```python
from build123d import *

# Parameters (mm, degrees)
SKETCH1_R           = 35
SKETCH1_R_2         = 15
BOSS_EXTRUDE1_DEPTH = 10
SKETCH5_R           = 35
BOSS_EXTRUDE3_DEPTH = 10
SKETCH4_R           = 2.5
BOSS_EXTRUDE2_DEPTH = 2


with BuildPart() as part:
    # Sketch1 → Boss-Extrude1 (new body)
    with BuildSketch(Plane.XY):
        Circle(SKETCH1_R)
        Circle(SKETCH1_R_2, mode=Mode.SUBTRACT)
    extrude(amount=BOSS_EXTRUDE1_DEPTH)

    # Sketch2 for Loft1 → Loft1 section 0
    with BuildSketch(Plane(origin=(0, 0, 0), x_dir=(0, 0, -1), z_dir=(1, 0, 0))):
        with BuildLine():
            Line((-10, -20), (-2.996710384, -20))
            # circular arc as an exact rational Bezier (weights 1, cos(half-angle), 1)
            Bezier((-2.996710384, -20), (35, -55.538461538), (72.996710384, -20), weights=[1, 0.730337079, 1])
            Line((72.996710384, -20), (80, -20))
            Bezier((80, -20), (35, -69.846153846), (-10, -20), weights=[1, 0.670103093, 1])
        make_face()
    # Sketch3 for Loft1 → Loft1 section 1
    with BuildSketch(Plane(origin=(100, 0, 0), x_dir=(0, 0, -1), z_dir=(1, 0, 0))):
        with BuildLine():
            Line((10, -15), (6.551180448, -15))
            Bezier((6.551180448, -15), (40, -77.258592471), (73.448819552, -15), weights=[1, 0.47327653, 1])
            Line((73.448819552, -15), (70, -15))
            Bezier((70, -15), (40, -65.081833061), (10, -15), weights=[1, 0.513877208, 1])
        make_face()
    loft()

    # Sketch5 → Boss-Extrude3 (add)
    with BuildSketch(Plane.XY.offset(10)):
        with Locations(Location((0, 0, 0), (0, 0, 314.528269686))):
            Circle(SKETCH5_R)
    extrude(amount=BOSS_EXTRUDE3_DEPTH)

    # Sketch7 → Revolve1 (revolve)
    with BuildSketch(Plane.ZY, mode=Mode.PRIVATE) as revolve1_sk:
        with BuildLine():
            Line((20, 34), (20, 39))
            Line((20, 39), (17.5, 39))
            Line((17.5, 39), (16.153846154, 35.769230769))
            ThreePointArc((16.153846154, 35.769230769), (15, 35), (13.846153846, 35.769230769))
            Line((13.846153846, 35.769230769), (12.5, 39))
            Line((12.5, 39), (10, 39))
            Line((10, 39), (10, 34))
            Line((10, 34), (20, 34))
        make_face()
    revolve(revolve1_sk.sketch.rotate(Axis((0, 0, 20), (0, 0, -1)), 90), axis=Axis((0, 0, 20), (0, 0, -1)))

    # Sketch4 → Boss-Extrude2 (add)
    with BuildSketch(Plane.XY.offset(20)):
        with Locations((0, 25)):
            Circle(SKETCH4_R)
    extrude(amount=BOSS_EXTRUDE2_DEPTH)


solid = part.part
```
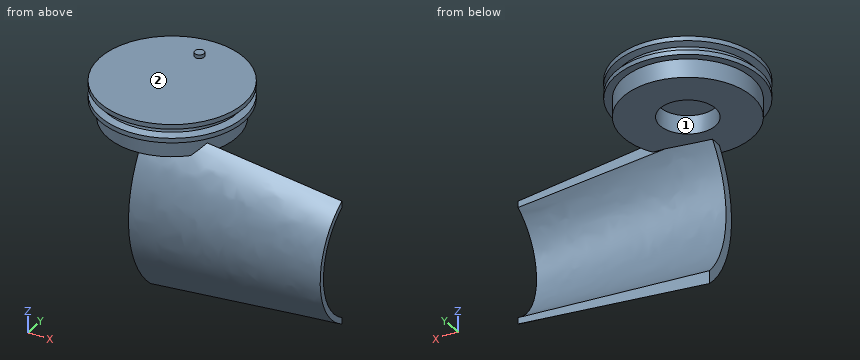
Can you work these out from the model? Positions are in its coordinate system, mm. Face numbers are marked on the shaded views. Coordinates: 2 decimals unless noted, no trailing zeros. Order: outer loops, then holes, each group sorted by start corner. A loop starts at its lowest first (then second) coordinate and runs counter-clockwise, first axis right, second up.
1. I need wall thicknesses on line 1 (Y direction, x = 0, z = 3.5); line 2 (Z direction, x = 9.5, y = 20); line 3 (Y direction, x = 35, z = -26). Which ranges of each line are inside material? Lowest first, please.
2. I'm going to push flat-ended pins straight in: pin 1 (23.5 mm diameter, centred on x = -8, y = 18.5, fed in from -Z); pin 2 (6 mm diameter, centred on y = -31.5, z = -44.5, fed in from -X); pin 3 (6 mm diameter, centred on x = 27, z = 10.5, fed in from -Y). Where does each tip first touch, or does it pass through?
3. If we section it at A-A (y = 0): Please give me the cut outline in (x, z).
4. Thinking about a two-plate mould opening in X: for the marked faces 1 and 2, which applies, +X half, -X half, draft (parallel to the pull), parting line (faces both ways), or undercut?
5. If we section it at B-B (z = 7): Please give me the cut outline in (x, y), then the cut area to 3 significant figures.
Entries:
1. line 1: y = -35 to -15, 15 to 35
1. line 2: z = 0 to 20
1. line 3: y = -37.12 to -32.71
2. pin 1: stops at z = 0
2. pin 2: stops at x = 0
2. pin 3: stops at y = -30.74
3. outline: (-39, 10) - (-35, 10) - (-35, 0) - (-15, 0) - (-15, 10) - (15, 10) - (15, 0) - (35, 0) - (35, 10) - (39, 10) - (39, 12.5) - (35.77, 13.85) arc R1.25 cw to (35.77, 16.15) - (39, 17.5) - (39, 20) - (-39, 20) - (-39, 17.5) - (-35.77, 16.15) arc R1.25 cw to (-35.77, 13.85) - (-39, 12.5) - close
4. face 1: undercut
4. face 2: draft
5. outline: circle Ø70 at (0, 0); hole circle Ø30 at (0, 0)
5. area: 3,140 mm2
